Drawing for the job (mm, zero at the part's lowest x, y, z). Round coordinates to 2 decimals unless told otherwise and drop trailing zeros. Write each loop counter-clockwise with the first axis right and the second up, starting at its lowest first coordinate (ties: lowest second). Pieces come first, ordered by that corner, then holes. Notation, with made-up numbers: (73.5, 69.5) - (127.5, 69.5) arc R18 ccw to (127.5, 94.5) - close; hole circle Ø8 at (23.5, 55). An arc over 180 degrees is marked (long way). Answer in a Markdown table with one row per item.
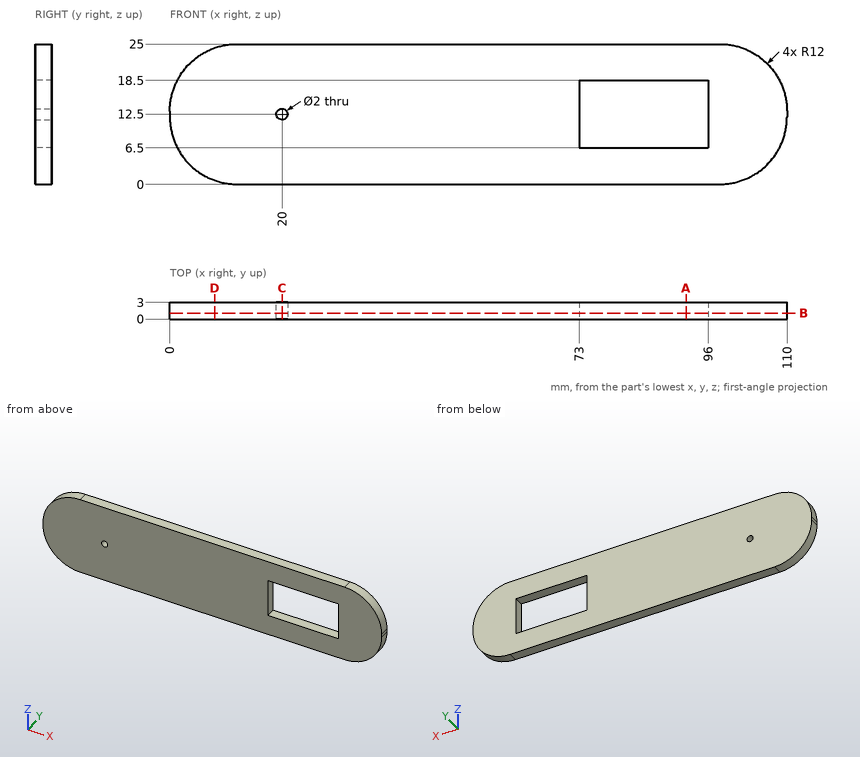
Q1. Saw through at A-A on x = 92. List the corners of the cut face in (y, z), then the cut area to 3 significant figures.
Computed:
| item | result |
|---|---|
| outline | (0, 0) - (3, 0) - (3, 6.5) - (0, 6.5) - close; (0, 18.5) - (3, 18.5) - (3, 25) - (0, 25) - close |
| area | 39.0 mm2 |
Q2. Flat gauge pins, fed straight in: pin 1 (1 mm diameter, centred on y = 2.5, z = 2.5, fed in from +X); pin 2 (1 mm diameter, centred on y = 1, z = 3.5, fed in from -X); pin 3 (1.5 mm diameter, centred on y = 0.5, z = 21.5, fed in from +X). Where does each tip first touch, or does it go through?
Computed:
| item | result |
|---|---|
| pin 1 | stops at x = 105.94 |
| pin 2 | stops at x = 3.06 |
| pin 3 | stops at x = 107.16 |
Q3. Saw through at D-D on x = 8. List the corners of the cut face in (y, z), then the cut area to 3 significant figures.
Computed:
| item | result |
|---|---|
| outline | (0, 0.69) - (3, 0.69) - (3, 24.31) - (0, 24.31) - close |
| area | 70.9 mm2 |
Q4. Saw through at B-B on y = 1.05. List the corners of the cut face in (x, z).
Computed:
| item | result |
|---|---|
| outline | (0, 12) arc R12 ccw to (12, 0) - (98, 0) arc R12 ccw to (110, 12) - (110, 13) arc R12 ccw to (98, 25) - (12, 25) arc R12 ccw to (0, 13) - close; hole circle Ø2 at (20, 12.5); hole (73, 6.5) - (96, 6.5) - (96, 18.5) - (73, 18.5) - close |
Q5. Drill centre lines: line 1 (X direction, y = 0.85, z = 12.5); line 2 (Z direction, x = 20, y = 1.35); line 3 (Z direction, x = 81, y = 0.8). Where is each one in solid material? Low to high.
Computed:
| item | result |
|---|---|
| line 1 | x = 0 to 19, 21 to 73, 96 to 110 |
| line 2 | z = 0 to 11.5, 13.5 to 25 |
| line 3 | z = 0 to 6.5, 18.5 to 25 |
Q6. Saw through at C-C on x = 20. List the corners of the cut face in (y, z).
Computed:
| item | result |
|---|---|
| outline | (0, 0) - (3, 0) - (3, 11.5) - (0, 11.5) - close; (0, 13.5) - (3, 13.5) - (3, 25) - (0, 25) - close |
